Could you check a few things on this model? Use its own coordinates, in mm. Give positions to 0.01 mm unless a question says otherwise; leave off trailing zeros. Write each loop counter-clockwise with the first axis right and the second up, starting at its lowest first coordinate (ties: lowest second). Pieces come first, ordered by that corner, then holes. Notation, with made-up numbers: M 50,-33.5 L 61,-33.5 A22 ccw 61,-10.5 Z; hole C -2,68 d3. An arc over 180 degrees is marked long. Use one line per item in the form item = value.
from build123d import *

# Parameters (mm, degrees)
SKETCH1_W           = 60
SKETCH1_H           = 50
BOSS_EXTRUDE1_DEPTH = 5
SKETCH2_R           = 6
SKETCH2_R_2         = 1.5
CUT_EXTRUDE1_DEPTH  = 5
FILLET1_R           = 5


with BuildPart() as part:
    # Sketch1 → Boss-Extrude1 (new body)
    with BuildSketch(Plane(origin=(0, 0, 0), x_dir=(1, 0, 0), z_dir=(0, 1, 0))):
        Rectangle(SKETCH1_W, SKETCH1_H)
    extrude(amount=BOSS_EXTRUDE1_DEPTH)

    # Sketch2 → Cut-Extrude1 (cut)
    with BuildSketch(Plane(origin=(0, 5, 0), x_dir=(1, 0, 0), z_dir=(0, 1, 0))):
        with Locations(Location((0, 7, 0), (0, 0, 270))):
            Circle(SKETCH2_R)
        with Locations(Location((-7.75, 13.423393759, 0), (0, 0, 270))):
            Circle(SKETCH2_R_2)
        with Locations(Location((-15.5, 0, 0), (0, 0, 270))):
            Circle(SKETCH2_R_2)
        with Locations(Location((-7.75, -13.423393759, 0), (0, 0, 270))):
            Circle(SKETCH2_R_2)
        with Locations(Location((7.75, -13.423393759, 0), (0, 0, 270))):
            Circle(SKETCH2_R_2)
        with Locations(Location((15.5, 0, 0), (0, 0, 270))):
            Circle(SKETCH2_R_2)
        with Locations(Location((7.75, 13.423393759, 0), (0, 0, 270))):
            Circle(SKETCH2_R_2)
        with Locations(Location((-20, 22.5, 0), (0, 0, 270))):
            Circle(SKETCH2_R_2)
        with Locations(Location((20, 22.5, 0), (0, 0, 270))):
            Circle(SKETCH2_R_2)
        with Locations(Location((20, -22.5, 0), (0, 0, 270))):
            Circle(SKETCH2_R_2)
        with Locations(Location((-20, -22.5, 0), (0, 0, 270))):
            Circle(SKETCH2_R_2)
        with Locations(Location((-27.5, 0, 0), (0, 0, 270))):
            Circle(SKETCH2_R_2)
        with Locations(Location((27.5, 0, 0), (0, 0, 270))):
            Circle(SKETCH2_R_2)
    extrude(amount=-CUT_EXTRUDE1_DEPTH, mode=Mode.SUBTRACT)

    # Fillet1
    fillet1_edges = [part.edges().sort_by_distance(p)[0] for p in [
        (30, 2.5, 25),
        (-30, 2.5, 25),
        (-30, 2.5, -25),
        (30, 2.5, -25),
    ]]
    fillet(fillet1_edges, radius=FILLET1_R)


solid = part.part
1) Thinking about a two-plate mould opening in Z: for faces 1 (the cylindrical face through (-26, 3, 0)), 2 (the flat face through (0, 0, 0)), 3 (the cylindrical face through (28, 3, -24)), which applies, released by +Z, released by -Z, zero draft, split by the parting line, or undercut?
Checked values:
face_1 = undercut
face_2 = zero draft
face_3 = released by -Z
2) I want a section at D-D, the plane z = 0. Please give me the cut outline in (x, y).
Checked values:
outline = M -30,0 L -29,0 L -29,5 L -30,5 Z; M -26,0 L -17,0 L -17,5 L -26,5 Z; M -14,0 L 14,0 L 14,5 L -14,5 Z; M 17,0 L 26,0 L 26,5 L 17,5 Z; M 29,0 L 30,0 L 30,5 L 29,5 Z
3) I want a section at C-C, the plane x = 0. Please give me the cut outline in (y, z).
Checked values:
outline = M 0,-25 L 5,-25 L 5,-13 L 0,-13 Z; M 0,-1 L 5,-1 L 5,25 L 0,25 Z
4) For pin 1 Ø2.5 at (x, z) = (-27.5, 0) entering from -Y, with a flat end and sliding along its axis, tell me the tip position at first contact or that it passes through.
Checked values:
pin_1 = through
5) I want a section at A-A, the plane z = -7. Please give me the cut outline in (x, y).
Checked values:
outline = M -30,0 L -6,0 L -6,5 L -30,5 Z; M 6,0 L 30,0 L 30,5 L 6,5 Z
6) I want a section at B-B, the plane y = 3.7. Count the separate pieces of the cut face and the enclosed holes in it, plus the area to 3 significant figures.
Checked values:
separate_pieces = 1
enclosed_holes = 13
area = 2,780 mm2
7) If I drill on L1, parallel to X at y = 3.2, z = 13.5; L2, parallel to X at y = 3.75, z = 0; L3, parallel to X at y = 3.4, z = -7, over which ranges is the centre line in solid material (lowest first)?
Checked values:
L1 = -30 to -9.25, -6.25 to 6.25, 9.25 to 30
L2 = -30 to -29, -26 to -17, -14 to 14, 17 to 26, 29 to 30
L3 = -30 to -6, 6 to 30
